Geometry check sheet. Reference: drawing and pictorial views, mm from the part's lowest x, y, z. A direction names the side the tool comes from. Give positions to 0.01 mm unless a question says otherwise; leave off trailing zeros. Order: outer loops, then holes, each group sorted by start corner. A loop starts at its lowest first (then second) coordinate and runs counter-clockwise, first axis right, second up. Notation, with made-up numbers: (17, -31.75) - (70, -31.75) arc R13 ccw to (70, -25.75) - close; hole circle Ø4 at (14, 79.25). An arc over 180 degrees is marked (long way). Answer in a Markdown table with one row per item.
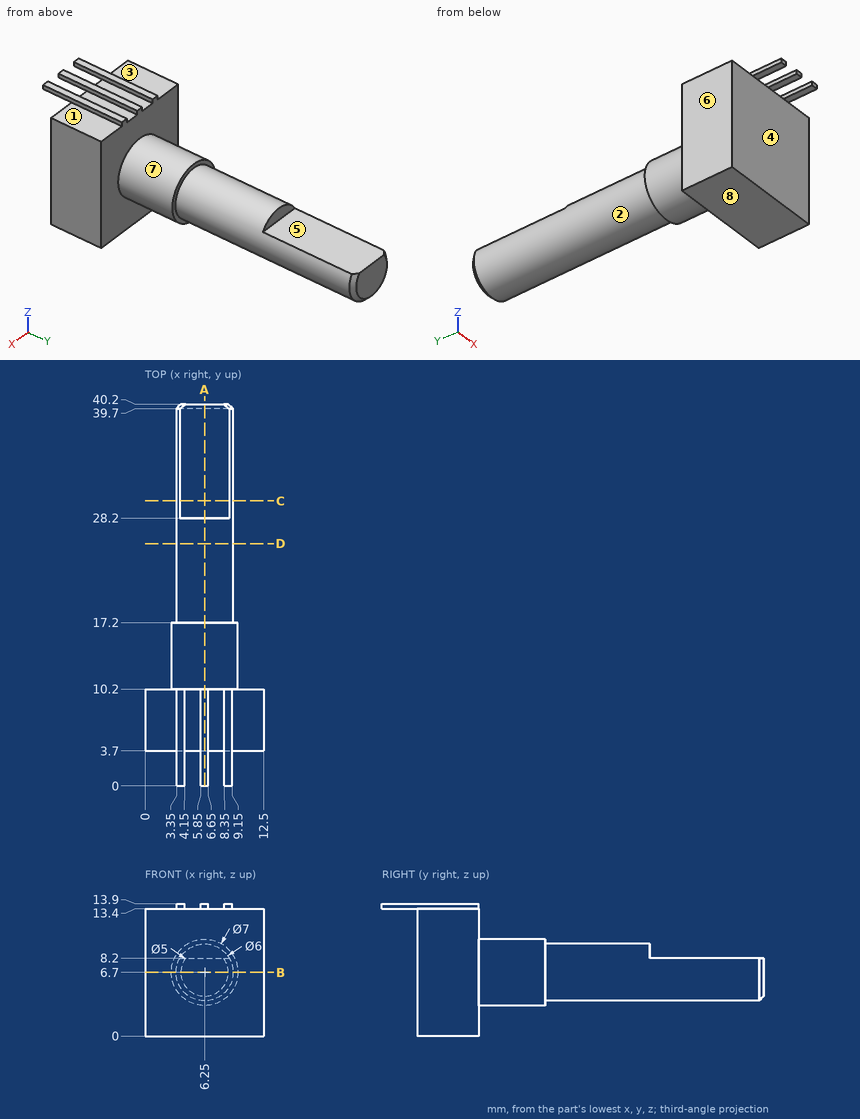
(1) Gauge pin test, flat ends, axial feed: P1, Ø6, axis at y = 16.5, z = 1.5, coming from the -X side; P2, Ø2.5, axis at x = 11, y = 6, coming from the +Z side; P3, Ø6, axis at y = 33, z = 5.5, coming from the -X side. Record the tip position at first contact, or that the pin passes through.
Geometry says:
| item | result |
|---|---|
| P1 | x = 3.53 |
| P2 | z = 13.4 |
| P3 | x = 3.25 |
(2) Cross-section at C-C, the plane y = 30. Record the cut outline in (x, z).
Geometry says:
| item | result |
|---|---|
| outline | (3.65, 8.2) arc R3 ccw (long way) to (8.85, 8.2) - close |
(3) Access from +Z, -Z, +X, -X, +Y, -Y to the whole of each face (thin tool, end or side, straight path). Record for the marked faces 1, 2, 3 and 4.
Geometry says:
| item | result |
|---|---|
| face 1 | +Z, +X, +Y, -Y |
| face 2 | +Y |
| face 3 | +Z, -X, +Y, -Y |
| face 4 | -Z, +X, -X, -Y |
(4) Cross-section at B-B, the plane z = 6.7. Record the cut outline in (x, y), then the cut area to 3 significant figures.
Geometry says:
| item | result |
|---|---|
| outline | (0, 3.7) - (12.5, 3.7) - (12.5, 10.2) - (9.75, 10.2) - (9.75, 17.2) - (9.25, 17.2) - (9.25, 39.7) - (8.75, 40.2) - (3.75, 40.2) - (3.25, 39.7) - (3.25, 17.2) - (2.75, 17.2) - (2.75, 10.2) - (0, 10.2) - close |
| area | 268 mm² |
(5) Cross-section at D-D, the plane y = 25.5. Record the cut outline in (x, z), then the cut area to 3 significant figures.
Geometry says:
| item | result |
|---|---|
| outline | circle Ø6 at (6.25, 6.7) |
| area | 28.3 mm² |
(6) Thickness scan on L1, parallel to Y at x = 11.75, z = 0.75; L2, parallel to Y at x = 4, z = 6.25; L3, parallel to Z at x = 5.5, y = 9. Record the ranges inside material, lowest first.
Geometry says:
| item | result |
|---|---|
| L1 | 3.7 to 10.2 |
| L2 | 3.7 to 40.2 |
| L3 | 0 to 13.4 |
(7) Cross-section at A-A, the plane x = 6.25. Record the cut outline in (y, z), then the cut area to 3 significant figures.
Geometry says:
| item | result |
|---|---|
| outline | (0, 13.4) - (3.7, 13.4) - (3.7, 0) - (10.2, 0) - (10.2, 3.2) - (17.2, 3.2) - (17.2, 3.7) - (39.7, 3.7) - (40.2, 4.2) - (40.2, 8.2) - (28.2, 8.2) - (28.2, 9.7) - (17.2, 9.7) - (17.2, 10.2) - (10.2, 10.2) - (10.2, 13.9) - (0, 13.9) - close |
| area | 261 mm² |
(8) Mould release check, pull along Z, two halves, no side actions. Record for the marked faces 5, 6, 7 and 8: pulls with the +Z half, pulls with the -Z half, needs draft (parallel to the pull), parting line crosses it, or undercut.
Geometry says:
| item | result |
|---|---|
| face 5 | pulls with the +Z half |
| face 6 | needs draft |
| face 7 | parting line crosses it |
| face 8 | pulls with the -Z half |
